The listing builds one solid part. Answer for the finished solid, in the listing's coordinates (mm). A direction names the side the tool comes from. Coordinates: 2 decimals unless noted, no trailing zeros. Loops run counter-clockwise (first coordinate to the right, second up) from the corner with the lowest first, then second, coordinate; pieces in that order, holes last. Notation, with made-up numbers: M 56.5,-34 L 79.5,-34 A27 ccw 79.5,-1 Z; hole C 46.25,-3.5 d7. An arc over 180 degrees is marked long. Return JSON: item names as keys, results as strings. Group by question number.
1. Given P1, Ø6, axis at y = -16.5, z = 8.5, coming from the +X side; P2, Ø5, axis at x = -15, z = 6, coming from the -Y side; P3, Ø1.5, axis at x = -36.5, z = 1, coming from the -Y side; P4, Ø3.5, axis at y = -38, z = 2, coming from the -X side, each flat-ended and moving along its own axis, determine where each tip first touches the part or whether it passes through.
2. Section A-A (y = -15) is taken. Write down the section's boundary in (x, z), then the cut area to 3 significant figures.
3. Section D-D (x = -4.5) is taken. Write down the section's boundary in (y, z).
4. The mould has two halves that part along Z. Classify faces 1 (the face through (-3, -31, 7)), 2 (the face through (-1, -15, 8)), 3 (the face through (-1, -17, 11)): pulls with the +Z half, pulls with the -Z half, needs draft (parallel to the pull), parting line crosses it, or undercut.
5. Which of the six approach directions +Z, -Z, +X, -X, +Y, -Y give full straight-line access (tool end or side, diameter ignored) to faces 4 (the face through (-13.526, -1.479, 7.352)), 5 (the face through (-21, -8, 3)), 6 (the face through (-35, -10, 1))?
6. Section C-C (z = 6) is taken. Write down the section's boundary in (x, y), then the cut area to 3 significant figures.
7. Straight lines are drawn through the part: L1, parallel to Z at x = -15, y = -1; L2, parallel to X at y = -29, z = 8.5; L3, parallel to Y at x = -2.5, z = 7.5. For each, find the intervals that lie inside material, in ascending order. Write a range as from..to.
```python
from build123d import *

# Parameters (mm, degrees)
F1_DEPTH = 3
F3_DEPTH = 8
F4_R     = 2
F5_DEPTH = 4
F6_R     = 2
F7_DEPTH = 6


with BuildPart() as f1:
    # F0 (on Top) → F1 (new body)
    with BuildSketch(Plane.XY):
        Polygon((0, 0), (-60, 0), (-60, -10), (-10, -10), (-10, -60), (0, -60), align=None)
    extrude(amount=F1_DEPTH)

    # F2 (on face) → F3 (join)
    with BuildSketch(Plane.XY.offset(3)):
        Polygon((0, 0), (-60, 0), (-60, -3), (-3, -3), (-3, -60), (0, -60), align=None)
    extrude(amount=F3_DEPTH)

    # F4 (on face) → F5 (cut)
    with BuildSketch(Plane.YZ):
        with Locations((-15, 6)):
            Circle(F4_R)
        with Locations((-45, 6)):
            Circle(F4_R)
    extrude(amount=-F5_DEPTH, mode=Mode.SUBTRACT)

    # F6 (on face) → F7 (cut)
    with BuildSketch(Plane(origin=(0, 0, 0), x_dir=(-1, 0, 0), z_dir=(0, 1, 0))):
        with Locations((45, 6)):
            Circle(F6_R)
        with Locations((15, 6)):
            Circle(F6_R)
    extrude(amount=-F7_DEPTH, mode=Mode.SUBTRACT)


solid = f1.part
```
Worked out:
{
 "1": {"P1": "x = 0", "P2": "y = -3", "P3": "y = -10", "P4": "x = -10"},
 "2": {"outline": "M -10,0 L 0,0 L 0,4 L -3,4 L -3,3 L -10,3 Z; M -3,8 L 0,8 L 0,11 L -3,11 Z", "area": "42.0 mm^2"},
 "3": {"outline": "M -60,0 L 0,0 L 0,11 L -3,11 L -3,3 L -60,3 Z"},
 "4": {"face 1": "needs draft", "face 2": "undercut", "face 3": "pulls with the +Z half"},
 "5": {"face 4": "+Y, -Y", "face 5": "+Z, -X, -Y", "face 6": "+Z, -Z, -X, -Y"},
 "6": {"outline": "M -60,-3 L -47,-3 L -47,0 L -60,0 Z; M -43,-3 L -17,-3 L -17,0 L -43,0 Z; M -13,-3 L -3,-3 L -3,-13 L 0,-13 L 0,0 L -13,0 Z; M -3,-60 L 0,-60 L 0,-47 L -3,-47 Z; M -3,-43 L 0,-43 L 0,-17 L -3,-17 Z", "area": "303 mm^2"},
 "7": {"L1": "0..4, 8..11", "L2": "-3..0", "L3": "-60..-46.32, -43.68..-16.32, -13.68..0"}
}
